The listing builds one solid part. Answer for the finished solid, in the listing's coordinates (mm). A direction names the side the tool comes from. Give positions to 0.01 mm unless a question says otherwise; leave off trailing zeros. Write each loop counter-clockwise with the first axis right and the second up, starting at its lowest first coordinate (ties: lowest second). Pieces come first, ordered by that corner, then holes. Notation, with made-up numbers: M -6,7 L 50,7 A22 ccw 50,28 Z; hole C 77,33.25 d10. An arc over 180 degrees is marked long. Answer as a JSON object with one key per item and string values.
Autodesk Inventor part; units mm, degrees
ref_plane "YZ Plane" through (0, 0, 0) normal (1, 0, 0) x (0, 1, 0)
ref_plane "XZ Plane" through (0, 0, 0) normal (0, 1, 0) x (-1, 0, 0)
ref_plane "XY Plane" through (0, 0, 0) normal (0, 0, 1) x (1, 0, 0)
sketch "Sketch1" plane through (0, 0, 0) normal (0, 1, 0) x (-1, 0, 0)
  line L0 (-7.3323, 0) -> (-3.6662, 6.35)
  line L1 (-3.6662, 6.35) -> (3.6662, 6.35)
  line L2 (3.6662, 6.35) -> (7.3323, 0)
  line L3 (7.3323, 0) -> (3.6662, -6.35)
  line L4 (3.6662, -6.35) -> (-3.6662, -6.35)
  line L5 (-3.6662, -6.35) -> (-7.3323, 0)
  point P0 (0, 0)
  point P1 (0, 0)
  dimension "d0" = 12.7
extrude "Extrusion1" add sketch "Sketch1" along normal blind 155.8036
sketch "Sketch2" plane through (0, 155.8036, 0) normal (0, 1, 0) x (1, 0, 0)
  circle A0 centre (0, 0) radius 2.5527
  dimension "d3" = 5.1054
sketch "Sketch3" plane through (0, 0, 0) normal (0, -1, 0) x (1, 0, 0)
  circle A0 centre (0, 0) radius 2.5527
  dimension "d4" = 5.1054
extrude "Extrusion2" cut sketch "Sketch3" against normal blind 25.4
extrude "Extrusion3" cut sketch "Sketch2" against normal blind 25.4
properties part number "INDX_016_BottomHex" material "Aluminum 6061"
1. Consider line 1 along Z through (x, y) = (0, 11.75); line 2 along X through (y, z) = (148, 0); line 3 along X through (y, z) = (23.5, -1.75). Determine where each line is inside the solid, lowest interval first.
Verdict:
{"line 1": "z = -6.35 to -2.55, 2.55 to 6.35", "line 2": "x = -7.33 to -2.55, 2.55 to 7.33", "line 3": "x = -6.32 to -1.86, 1.86 to 6.32"}
2. A cutting plane is placed at C-C, the plane y = 106.5. Give the vertices of the cut face in (x, z).
Verdict:
{"outline": "M -7.33,0 L -3.67,-6.35 L 3.67,-6.35 L 7.33,0 L 3.67,6.35 L -3.67,6.35 Z"}
3. Flat-ended cylindrical pins translate along their axes: pin 1 (2 mm diameter, centred on y = 128, z = -5, fed in from +X); pin 2 (6 mm diameter, centred on x = 0, z = 0, fed in from -Y); pin 3 (1 mm diameter, centred on x = 0, z = -1.5, fed in from -Y); pin 4 (4 mm diameter, centred on y = 20, z = 1, fed in from -X). Find the tip coordinate at first contact, or state that the pin passes through.
Verdict:
{"pin 1": "stops at x = 5.02", "pin 2": "stops at y = 0", "pin 3": "stops at y = 25.4", "pin 4": "stops at x = -7.33"}
4. For faces 1 (the cylindrical face through (2.435, 12.522, 0.767)), 2 (the flat face through (0, 130.404, 0)), 3 (the flat face through (5.525, 76.811, 3.131)), determine the directions among +Z, -Z, +X, -X, +Y, -Y from which every point of the face is accessible in a straight line to the end or side of a thin tool.
Verdict:
{"face 1": "-Y", "face 2": "+Y", "face 3": "+Z, +X, +Y, -Y"}
5. A cutting plane is placed at B-B, the plane x = 0. Give the vertices of the cut face in (y, z), plus the area to 3 significant figures.
Verdict:
{"outline": "M 0,-6.35 L 155.8,-6.35 L 155.8,-2.55 L 130.4,-2.55 L 130.4,2.55 L 155.8,2.55 L 155.8,6.35 L 0,6.35 L 0,2.55 L 25.4,2.55 L 25.4,-2.55 L 0,-2.55 Z", "area": "1,720 mm2"}
6. The mould has two halves that part along Z. Classify faces 4 (the flat face through (0, 77, 6.35)), 5 (the cylindrical face through (2.435, 143.281, -0.767)), 6 (the flat face through (5.474, 76.811, -3.219)): released by +Z, released by -Z, zero draft, split by the parting line, or undercut.
Verdict:
{"face 4": "released by +Z", "face 5": "undercut", "face 6": "released by -Z"}
7. A cutting plane is placed at A-A, the plane y = 143. Give the vertices of the cut face in (x, z).
Verdict:
{"outline": "M -7.33,0 L -3.67,-6.35 L 3.67,-6.35 L 7.33,0 L 3.67,6.35 L -3.67,6.35 Z; hole C 0,0 d5.11"}
8. A cutting plane is placed at D-D, the plane z = -4.75. Give the vertices of the cut face in (x, y), plus the area to 3 significant figures.
Verdict:
{"outline": "M -4.59,0 L 4.59,0 L 4.59,155.8 L -4.59,155.8 Z", "area": "1,430 mm2"}
